Source: CAD feature listing. Evaluate the final solid. Frame: model axes, mm. Give positions to 0.01 mm unless a question says otherwise; leave off trailing zeros. Write each loop counter-clockwise with the first axis right and the second up, starting at its lowest first coordinate (ties: lowest second). Pieces come first, ordered by that corner, then holes. Notation, with made-up numbers: (-10, 58.25) - (34, 58.25) arc R16 cw to (34, 67.25) - close; hole circle Ø3 at (3, 63.25). An arc over 180 degrees is marked (long way). Answer as a JSON object with one key per item and string values. Group by question number.
Autodesk Inventor part; units mm, degrees
ref_plane "YZ Plane" through (0, 0, 0) normal (1, 0, 0) x (0, 1, 0)
ref_plane "XZ Plane" through (0, 0, 0) normal (0, 1, 0) x (-1, 0, 0)
ref_plane "XY Plane" through (0, 0, 0) normal (0, 0, 1) x (1, 0, 0)
sketch "Esquisse1" plane through (0, 0, 0) normal (0, 0, 1) x (1, 0, 0)
  line L0 (0, 89) -> (85, 89)
  line L1 (85, 89) -> (85, 0)
  line L2 (85, 0) -> (0, 0)
  line L3 (0, 0) -> (0, 89)
  line L4 (-17.3397, 0) -> (102.0566, 0)
  line L5 (0, -18.665) -> (0, 106.9442)
  point P0 (0, 0)
  dimension "d0" = 85
  dimension "d1" = 89
extrude "Extrusion1" add sketch "Esquisse1" along normal blind 4
sketch "Esquisse2" plane through (0, 0, 4) normal (0, 0, 1) x (1, 0, 0)
  line L0 (85, 0) -> (85, 89)
  line L1 (0, 89) -> (0, 0)
  line L2 (85, 89) -> (0, 89)
  line L3 (0, 0) -> (85, 0)
  point P0 (5, 84)
  point P1 (80, 84)
  point P2 (80, 5)
  point P3 (5, 5)
  dimension "d16" = 75
  dimension "d17" = 75
  dimension "d18" = 79
  dimension "d19" = 79
  dimension "d20" = 5
  dimension "d21" = 5
  dimension "d22" = 5
  dimension "d23" = 5
hole "Perçage1" at (5, 84, 4) at (80, 84, 4) at (80, 5, 4) at (5, 5, 4) direction (0, 0, -1) diameter 2.5 end through all
sketch "Esquisse3" plane through (0, 0, 0) normal (0, 0, -1) x (-1, 0, 0)
  line L0 (0, 0) -> (0, 89)
  line L1 (0, 89) -> (-85, 89)
  point P0 (-21, 66)
  point P1 (-21, 23)
  point P2 (-64, 23)
  point P3 (-64, 66)
  dimension "d32" = 43
  dimension "d33" = 43
  dimension "d34" = 43
  dimension "d35" = 43
  dimension "d36" = 21
  dimension "d44" = 21
  dimension "d45" = 23
  dimension "d46" = 23
hole "Perçage2" at (21, 66, 0) at (21, 23, 0) at (64, 23, 0) at (64, 66, 0) direction (0, 0, 1) diameter 2 end through all
chamfer "Chanfrein1" distance 1 angle 45 8 edges at (42.5, 0, 0) (42.5, 0, 4) (85, 44.5, 0) (42.5, 89, 0) (0, 44.5, 0) (0, 44.5, 4) (85, 44.5, 4) (42.5, 89, 4)
properties part number "support lidar"
Q1. First-contact query: pin 1 Ø2 at (x, y) = (80, 84) entering from -Z. Flat tip, straight axial feed; report the tip coordinate or a pass-through.
Q2. Ray query, probe 1 along X at (y, z) = (23, 1.9); probe 2 along Y at (x, z) = (80, 1.75); probe 3 along X at (y, z) = (5, 2.3). Return the intervals inside material, ascending. Write a range as [from, to].
Q3. Section A-A on x = 5. Return the cut outline in (y, z).
Q4. Draft query along Y for faces 1 (the flat face through (42, 89, 2)), 2 (the flat face through (42, 45, 0)), 3 (the cylindrical face through (5.479, 82.845, 1.972)). Return one class per face: released by +Y, released by -Y, zero draft, split by the parting line, or undercut.
Q5. Section B-B on y = 5. Return the cut outline in (x, z), then the cut area to 3 significant figures.
Taken from the geometry:
{
 "1": {"pin 1": "passes through"},
 "2": {"probe 1": "x = [0, 20], [22, 63], [65, 85]", "probe 2": "y = [0, 3.75], [6.25, 82.75], [85.25, 89]", "probe 3": "x = [0, 3.75], [6.25, 78.75], [81.25, 85]"},
 "3": {"outline": "(0, 1) - (1, 0) - (3.75, 0) - (3.75, 4) - (1, 4) - (0, 3) - close; (6.25, 0) - (82.75, 0) - (82.75, 4) - (6.25, 4) - close; (85.25, 0) - (88, 0) - (89, 1) - (89, 3) - (88, 4) - (85.25, 4) - close"},
 "4": {"face 1": "released by +Y", "face 2": "zero draft", "face 3": "undercut"},
 "5": {"outline": "(0, 1) - (1, 0) - (3.75, 0) - (3.75, 4) - (1, 4) - (0, 3) - close; (6.25, 0) - (78.75, 0) - (78.75, 4) - (6.25, 4) - close; (81.25, 0) - (84, 0) - (85, 1) - (85, 3) - (84, 4) - (81.25, 4) - close", "area": "318 mm²"}
}
